Source: CAD feature listing. Evaluate the final solid. Frame: model axes, mm. A direction names the side the tool comes from. Give positions to 0.01 mm unless a question says otherwise; leave off trailing zeros. Loops run counter-clockwise (first coordinate to the right, second up) from the corner with the lowest first, then second, coordinate; pieces in that order, holes last.
Autodesk Inventor part; units mm, degrees
ref_plane "YZ Plane" through (0, 0, 0) normal (1, 0, 0) x (0, 1, 0)
ref_plane "XZ Plane" through (0, 0, 0) normal (0, 1, 0) x (-1, 0, 0)
ref_plane "XY Plane" through (0, 0, 0) normal (0, 0, 1) x (1, 0, 0)
sketch "Skizze1" plane through (0, 0, 0) normal (0, 0, 1) x (1, 0, 0)
  line L0 (0, -19.95) -> (0, 19.95) construction
  arc A0 (-5.5, -19.95) -> (5.5, -19.95) centre (0, -19.95) ccw
  arc A1 (5.5, 19.95) -> (-5.5, 19.95) centre (0, 19.95) ccw
  line L1 (0, 37.03) -> (0, -37.03) construction
  line L2 (-16.45, 0) -> (16.45, 0) construction
  circle A2 centre (0, 19.95) radius 1.5
  circle A3 centre (0, -19.95) radius 1.5
  circle A4 centre (0, 19.95) radius 6.5 construction
  circle A5 centre (0, -19.95) radius 6.5 construction
  line L3 (0, 26.45) -> (0, -26.45) construction
  circle A6 centre (0, 19.95) radius 2.5
  circle A7 centre (0, -19.95) radius 2.5
  circle A8 centre (0, 0) radius 9.75
  line L4 (-5.5, 19.95) -> (-5.5, 10.3833)
  line L5 (-5.5, -10.3833) -> (-5.5, -19.95)
  line L6 (5.5, -19.95) -> (5.5, -10.3833)
  line L7 (5.5, 10.3833) -> (5.5, 19.95)
  arc A9 (5.5, -10.3833) -> (5.5, 10.3833) centre (0, 0) ccw
  arc A10 (-5.5, 10.3833) -> (-5.5, -10.3833) centre (0, 0) ccw
  circle A11 centre (0, 0) radius 6.35 construction
  circle A12 centre (-4.4901, 4.4901) radius 1.5
  circle A13 centre (-4.4901, -4.4901) radius 1.5
  circle A14 centre (4.4901, -4.4901) radius 1.5
  circle A15 centre (4.4901, 4.4901) radius 1.5
  line L8 (-4.4901, 4.4901) -> (0, 0) construction
  dimension "d4" = 13
  dimension "d31" = 12.7
  dimension "d1" = 3
  dimension "d5" = 52.9
  dimension "d19" = 1
  dimension "d26" = 19.5
  dimension "d28" = 2
  dimension "d32" = 3
  dimension "d35" = 360
  dimension "d37" = 45
  dimension "d38" = 3
extrude "Extrusion1" add sketch "Skizze1" against normal blind 4 contours L5 A10 L4 A1 L7 A9 L6 A0 | A6 | A7
extrude "Extrusion4" add sketch "Skizze1" against normal blind 0.5 from surface at -4 contours A6 | A7
extrude "Extrusion6" add sketch "Skizze1" along normal blind 2 from surface at -4 contours A8
extrude "Extrusion7" add sketch "Skizze1" along normal blind 0.5 contours A6 | A7
properties part number "HarmonicDrive-WaveGenerator-Bottom"
1) Reachability of faces 4 (the flat face through (5.5, 15, -2)), 5 (the cylindrical face through (-1.269, 9.667, -0.986)), 6 (the cylindrical face through (1.15, -22.17, -4.25)) from +Z, -Z, +X, -X, +Y, -Y: full face, straight path, thin tool, end or side. Return the list, or none.
Checks:
face 4: +Z, -Z, +X, +Y
face 5: +Z
face 6: -Z
2) Cut plane C-C (y = 0). Return loops of the section in (x, z), and give its area (3 significant figures).
Checks:
outline: (-11.75, -4) - (11.75, -4) - (11.75, 0) - (9.75, 0) - (9.75, -2) - (-9.75, -2) - (-9.75, 0) - (-11.75, 0) - close
area: 55.0 mm2
3) Cut plane B-B (z = -0.5). Return loops of the section in (x, y).
Checks:
outline: (-5.5, -19.95) arc R5.5 ccw to (5.5, -19.95) - (5.5, -10.38) arc R11.75 ccw to (5.5, 10.38) - (5.5, 19.95) arc R5.5 ccw to (-5.5, 19.95) - (-5.5, 10.38) arc R11.75 ccw to (-5.5, -10.38) - close; hole circle Ø19.5 at (0, 0); hole circle Ø3 at (0, -19.95); hole circle Ø3 at (0, 19.95)
4) Ray query, probe 1 along Y at (x, z) = (0, -1.3); probe 2 along Y at (x, z) = (4.5, -2.65); probe 3 along Y at (x, z) = (3.5, -3.1). Return the intervals inside material, ascending.
Checks:
probe 1: y = -25.45 to -21.45, -18.45 to -9.75, 9.75 to 18.45, 21.45 to 25.45
probe 2: y = -23.11 to -5.99, -2.99 to 2.99, 5.99 to 23.11
probe 3: y = -24.19 to -5.62, -3.36 to 3.36, 5.62 to 24.19
5) Pull-direction query (Y, two-part tool) for faces 1 (the cylindrical face through (-0.5, -17.5, 0.2)), 2 (the cylindrical face through (0.12, 25.45, -1.97)), 3 (the flat face through (5.5, -15, -2)); classes: released by +Y, released by -Y, zero draft, split by the parting line, or undercut.
Checks:
face 1: undercut
face 2: released by +Y
face 3: zero draft
6) Contact query for flat-ended pins moving along their axis: P1, Ø1.5, axis at y = -11, z = -3.5, coming from the +X side; P2, Ø3, axis at y = -16, z = -1, coming from the +X side; P3, Ø1.5, axis at y = 7.5, z = -1.5, coming from the -X side. Output: stop coordinate, or through.
Checks:
P1: stops at x = 5.74
P2: stops at x = 5.5
P3: stops at x = -9.62
7) Cut plane D-D (x = 8.5). Return loops of the section in (y, z), and give its area (3 significant figures).
Checks:
outline: (-8.11, -4) - (8.11, -4) - (8.11, 0) - (4.78, 0) - (4.78, -2) - (-4.78, -2) - (-4.78, 0) - (-8.11, 0) - close
area: 45.8 mm2
8) Cut plane A-A (x = 0). State how many separate pieces and enclosed holes the cut face has, and give its area (3 significant figures).
Checks:
separate pieces: 3
enclosed holes: 0
area: 145 mm2
